from build123d import *

# Parameters (mm, degrees)
MAINBODY_DEPTH      = 6
HOOK_DEPTH          = 3.000005
FLEX_REACH          = 175.361
FLEX_END_RADIUS     = 12.225328947
SKETCH4_W           = 6.275
SKETCH4_H           = 8
FILLET1_R           = 1
FILLET2_R           = 1
SKETCH7_R           = 1.5
BOSS_EXTRUDE2_DEPTH = 5
FILLET3_R           = 1


with BuildPart() as part:
    # Sketch1 → MainBody (new, symmetric)
    with BuildSketch(Plane.XY):
        with BuildLine():
            Line((-159.798174106, 9.159375), (-172.248174106, 9.159375))
            Line((-172.248174106, 9.159375), (-172.248174106, -9.159375))
            Line((-172.248174106, -9.159375), (-159.798174106, -9.159375))
            Line((-159.798174106, -9.159375), (-159.798174106, -6.159375))
            ThreePointArc((-159.798174106, -6.159375), (-164.523174106, -5.209375), (-169.248174106, -6.159375))
            Line((-169.248174106, -6.159375), (-169.248174106, -5.159375))
            Line((-169.248174106, -5.159375), (-169.248174106, 5.159375))
            Line((-169.248174106, 5.159375), (-169.248174106, 6.159375))
            ThreePointArc((-169.248174106, 6.159375), (-164.523174106, 5.209375), (-159.798174106, 6.159375))
            Line((-159.798174106, 6.159375), (-159.798174106, 9.159375))
        make_face()
    extrude(amount=MAINBODY_DEPTH, both=True)

    # Sketch3 → Hook (add)
    with BuildSketch(Plane.XZ.offset(9.159375)):
        Polygon((-159.798174106, -6), (-161.898174106, -7), (-161.898174106, -6), align=None)
        Polygon((-161.898174106, 6), (-159.798174106, 6), (-161.898174106, 7), align=None)
    extrude(amount=-HOOK_DEPTH)

    # Flex: up to this cylinder (the profile starts inside it)
    flex_end = Plane(origin=(-164.523174106, -17.434703947, 0), z_dir=(0, 0, -1)) * Cylinder(FLEX_END_RADIUS, 376.172657895, mode=Mode.PRIVATE)
    # Sketch4 → Flex (cut, up to the surface)
    with BuildSketch(Plane.XZ.offset(9.159375), mode=Mode.PRIVATE) as flex_sk1:
        with Locations((-162.935674106, 0)):
            Rectangle(SKETCH4_W, SKETCH4_H)
    flex_tool1 = extrude(flex_sk1.sketch, amount=-FLEX_REACH, mode=Mode.PRIVATE) & flex_end
    add(flex_tool1.solids().sort_by_distance((-162.935674, -9.159375, 0))[0], mode=Mode.SUBTRACT)

    # Fillet1
    fillet1_edges = [part.edges().sort_by_distance(p)[0] for p in [
        (-166.073174106, -7.233703596, 4),
        (-166.073174106, -7.233703596, -4),
    ]]
    fillet(fillet1_edges, radius=FILLET1_R)

    # Fillet2
    fillet2_edges = [part.edges().sort_by_distance(p)[0] for p in [
        (-169.248174106, 6.159375, 0),
        (-169.248174106, -6.159375, 0),
    ]]
    fillet(fillet2_edges, radius=FILLET2_R)

    # Sketch7 → Boss-Extrude2 (add)
    with BuildSketch(Plane.ZY.offset(172.248174106)):
        with Locations(Location((0, 0, 0), (0, 0, 180))):
            Circle(SKETCH7_R)
    extrude(amount=BOSS_EXTRUDE2_DEPTH)

    # Fillet3
    fillet3_edges = [part.edges().sort_by_distance(p)[0] for p in [
        (-172.248174106, 0, 1.5),
    ]]
    fillet(fillet3_edges, radius=FILLET3_R)


solid = part.part
Check sheet for the modelled part. Datum: model origin and axes. Units: mm. A direction names the side the tool comes from. Round coordinates to 2 decimals unless told otherwise and drop trailing zeros. Loops run counter-clockwise (first coordinate to the right, second up) from the corner with the lowest first, then second, coordinate; pieces in that order, holes last. Notation, with made-up numbers: (23, 9.5) -> (80, 9.5) arc R10 cw to (80, 20.5) -> close; hole circle Ø3 at (69.5, 39.25). An arc over 180 degrees is marked (long way). Put each result on its own line as item: value. Start each with the question number.
1. Section check D-D (z = 4.75). Enter the section's corners in (x, y).
2. Gauge pin test, flat ends, axial feed: pin 1 (6 mm diameter, centred on y = 3, z = -2.5, fed in from -X); pin 2 (3 mm diameter, centred on y = -7.5, z = -1, fed in from +X); pin 3 (0.5 mm diameter, centred on y = -8, z = -6.5, fed in from -X); pin 4 (1.5 mm diameter, centred on x = -170, y = -0.5, fed in from -Z). Record the tip position at first contact, or that the pin passes through.
3. Draft check along Z on faces 1 (the face through (-160.83, -7.68, 6.49)), 2 (the face through (-165.79, -7.16, 3.7)), 3 (the face through (-166, 9.159, 0)). Enter one of: +Z half, -Z half, draft (parallel to the pull), parting line (faces both ways), or undercut.
4. Section check B-B (x = -170). Enter the section's corners in (y, z), plus the area to 3 significant figures.
5. Section check C-C (z = 0). Enter the section's corners in (x, y), plus the area to 3 significant figures.
6. Section check A-A (y = 0). Enter the section's corners in (x, z).
7. Access from +Z, -Z, +X, -X, +Y, -Y to the whole of each face (thin tool, end or side, straight path). Record for faces 4 (the face through (-165.772, -7.163, -3.715)), 5 (the face through (-172.248, 0, 3)), 6 (the face through (-163.901, 5.225, 0.084)), 7 (the face through (-161.3, -6.159, 6.3)).
8. Scan lines: probe 1 along Z at (x, y) = (-165, -8.5); probe 2 along X at (y, z) = (-7, 2); probe 3 along X at (y, z) = (3, 5.75). Record each from-to range of solid material in increasing order.
Findings:
1. outline: (-172.25, -9.16) -> (-159.8, -9.16) -> (-159.8, -6.16) arc R12.23 ccw to (-167.97, -5.7) arc R1 cw to (-169.25, -4.74) -> (-169.25, 4.74) arc R1 cw to (-167.97, 5.7) arc R12.23 ccw to (-159.8, 6.16) -> (-159.8, 9.16) -> (-172.25, 9.16) -> close
2. pin 1: stops at x = -177.25
2. pin 2: stops at x = -166.07
2. pin 3: stops at x = -161.9
2. pin 4: stops at z = -6
3. face 1: +Z half
3. face 2: undercut
3. face 3: draft
4. outline: (-9.16, -6) -> (9.16, -6) -> (9.16, 6) -> (-9.16, 6) -> close
4. area: 220 mm^2
5. outline: (-177.25, -1.5) -> (-173.25, -1.5) arc R1 cw to (-172.25, -2.5) -> (-172.25, -9.16) -> (-166.07, -9.16) -> (-166.07, -5.31) arc R12.23 ccw to (-167.97, -5.7) arc R1 cw to (-169.25, -4.74) -> (-169.25, 4.74) arc R1 cw to (-167.97, 5.7) arc R12.23 ccw to (-159.8, 6.16) -> (-159.8, 9.16) -> (-172.25, 9.16) -> (-172.25, 2.5) arc R1 cw to (-173.25, 1.5) -> (-177.25, 1.5) -> close
5. area: 117 mm^2
6. outline: (-177.25, -1.5) -> (-173.25, -1.5) arc R1 cw to (-172.25, -2.5) -> (-172.25, -6) -> (-169.25, -6) -> (-169.25, 6) -> (-172.25, 6) -> (-172.25, 2.5) arc R1 cw to (-173.25, 1.5) -> (-177.25, 1.5) -> close
7. face 4: +X, -Y
7. face 5: -X
7. face 6: +Z, -Z
7. face 7: +Z, +X, -X, +Y
8. probe 1: z = -6 to -4, 4 to 6
8. probe 2: x = -172.25 to -166.07
8. probe 3: x = -172.25 to -169.25
